Read the model definition and answer for the solid it produces. Units are mm, in the model's axes. Coordinates: 2 decimals unless noted, no trailing zeros. Loops run counter-clockwise (first coordinate to the right, second up) from the corner with the lowest first, then second, coordinate; pieces in that order, holes last.
Autodesk Inventor part; units mm, degrees
ref_plane "YZ Plane" through (0, 0, 0) normal (1, 0, 0) x (0, 1, 0)
ref_plane "XZ Plane" through (0, 0, 0) normal (0, 1, 0) x (-1, 0, 0)
ref_plane "XY Plane" through (0, 0, 0) normal (0, 0, 1) x (1, 0, 0)
sketch "Sketch1" plane through (0, 0, 0) normal (0, 0, 1) x (1, 0, 0)
  circle A0 centre (0, 51.9685) radius 11
  line L0 (21.15, 34.8185) -> (21.15, 69.1185)
  line L1 (21.15, 69.1185) -> (17.15, 73.1185)
  line L2 (17.15, 73.1185) -> (-17.15, 73.1185)
  line L3 (-17.15, 73.1185) -> (-21.15, 69.1185)
  line L4 (-21.15, 69.1185) -> (-21.15, 34.8185)
  line L5 (-21.15, 34.8185) -> (-17.15, 30.8185)
  line L6 (-17.15, 30.8185) -> (17.15, 30.8185)
  line L7 (17.15, 30.8185) -> (21.15, 34.8185)
  circle A1 centre (-15.5, 36.4685) radius 1.5
  circle A2 centre (15.5, 36.4685) radius 1.5
  circle A3 centre (15.5, 67.4685) radius 1.5
  circle A4 centre (-15.5, 67.4685) radius 1.5
  point P0 (0, 0)
extrude "Extrusion1" add sketch "Sketch1" along normal blind 2
properties part number "Stepper_spacer"
Q1. A flat-ended cylindrical pin translates along its axis: pin 1 Ø10 at (x, y) = (6.5, 56) entering from +Z. Find the tip coordinate at first contact, or state that the pin passes through.
Findings below:
pin 1: stops at z = 2
Q2. A cutting plane is placed at D-D (x = -15.5). Give the vertices of the cut face in (y, z), then the cut area to 3 significant figures.
Findings below:
outline: (30.82, 0) - (34.97, 0) - (34.97, 2) - (30.82, 2) - close; (37.97, 0) - (65.97, 0) - (65.97, 2) - (37.97, 2) - close; (68.97, 0) - (73.12, 0) - (73.12, 2) - (68.97, 2) - close
area: 72.6 mm2
Q3. A cutting plane is placed at B-B (y = 47.5). Give the vertices of the cut face in (x, z).
Findings below:
outline: (-21.15, 0) - (-10.05, 0) - (-10.05, 2) - (-21.15, 2) - close; (10.05, 0) - (21.15, 0) - (21.15, 2) - (10.05, 2) - close
Q4. Straight lines are drawn through the part: probe 1 along Y at (x, z) = (-15.5, 1.4); probe 2 along X at (y, z) = (35.5, 1.8); probe 3 along Y at (x, z) = (15, 0.35). For each, find the intervals that lie inside material, in ascending order.
Findings below:
probe 1: y = 30.82 to 34.97, 37.97 to 65.97, 68.97 to 73.12
probe 2: x = -21.15 to -16.65, -14.35 to 14.35, 16.65 to 21.15
probe 3: y = 30.82 to 35.05, 37.88 to 66.05, 68.88 to 73.12
Q5. Determine the mould class of faces 1 (the face through (-1.43, 41.06, 0.99)), 2 (the face through (-19.12, 71.15, 0.99)), 3 (the face through (15.17, 68.93, 0.99)), 4 (the face through (0, 73.118, 1)) for opening direction X: +X half, -X half, draft (parallel to the pull), parting line (faces both ways), or undercut.
Findings below:
face 1: undercut
face 2: -X half
face 3: undercut
face 4: draft
Q6. A cutting plane is placed at A-A (x = 0). Give the vertices of the cut face in (y, z), then the cut area to 3 significant figures.
Findings below:
outline: (30.82, 0) - (40.97, 0) - (40.97, 2) - (30.82, 2) - close; (62.97, 0) - (73.12, 0) - (73.12, 2) - (62.97, 2) - close
area: 40.6 mm2
Q7. A cutting plane is placed at C-C (z = 0.3). Give the vertices of the cut face in (x, y).
Findings below:
outline: (-21.15, 34.82) - (-17.15, 30.82) - (17.15, 30.82) - (21.15, 34.82) - (21.15, 69.12) - (17.15, 73.12) - (-17.15, 73.12) - (-21.15, 69.12) - close; hole circle Ø3 at (-15.5, 36.47); hole circle Ø3 at (-15.5, 67.47); hole circle Ø22 at (0, 51.97); hole circle Ø3 at (15.5, 36.47); hole circle Ø3 at (15.5, 67.47)
